from build123d import *

# Parameters (mm, degrees)
SKETCH013_W  = 32.5
SKETCH013_H  = 12.2
SKETCH013_R  = 1.35
PAD003_DEPTH = 1.2
SKETCH014_W  = 23
SKETCH014_H  = 12.2
PAD001_DEPTH = 1.4
PAD002_DEPTH = 6
SKETCH003_R  = 2.4
PAD005_DEPTH = 4.8
SKETCH016_W  = 23
SKETCH016_H  = 12.2
PAD004_DEPTH = 18.9
SKETCH012_W  = 3
SKETCH012_H  = 1
PAD008_DEPTH = 7


with BuildPart() as part:
    # Sketch013 → Pad003 (new body, symmetric)
    with BuildSketch(Plane.XY):
        Rectangle(SKETCH013_W, SKETCH013_H)
        with Locations((-13.8, 0)):
            Circle(SKETCH013_R, mode=Mode.SUBTRACT)
        with Locations((13.8, 0)):
            Circle(SKETCH013_R, mode=Mode.SUBTRACT)
    extrude(amount=PAD003_DEPTH, both=True)

    # Sketch014 → Pad001 (join)
    with BuildSketch(Plane.XY.offset(1.2)):
        Rectangle(SKETCH014_W, SKETCH014_H)
    extrude(amount=PAD001_DEPTH)

    # Sketch015 → Pad002 (join)
    with BuildSketch(Plane.XY.offset(2.6)):
        with BuildLine():
            ThreePointArc((-0.26712, 3.295988), (-11.5, 0), (-0.26712, -3.295988))
            ThreePointArc((0.490093, -2.839869), (0.058351, -2.979717), (-0.26712, -3.295988))
            ThreePointArc((0.490093, -2.839869), (3.1, 0), (0.490093, 2.839869))
            ThreePointArc((-0.26712, 3.295988), (0.058351, 2.979717), (0.490093, 2.839869))
        make_face()
    extrude(amount=PAD002_DEPTH)

    # Sketch003 → Pad005 (join)
    with BuildSketch(Plane.XY.offset(8.6)):
        with Locations((-5.4, 0)):
            Circle(SKETCH003_R)
    extrude(amount=PAD005_DEPTH)

    # Sketch016 → Pad004 (join)
    with BuildSketch(Plane(origin=(0, 0, -1.2), x_dir=(1, 0, 0), z_dir=(0, 0, -1))):
        Rectangle(SKETCH016_W, SKETCH016_H)
    extrude(amount=PAD004_DEPTH)

    # Sketch012 (on Face11 of Pad004) → Pad008 (join)
    with BuildSketch(Plane(origin=(-11.5, 0, 0), x_dir=(0, -1, 0), z_dir=(-1, 0, 0))):
        with Locations((0, -14.2)):
            Rectangle(SKETCH012_W, SKETCH012_H)
    extrude(amount=PAD008_DEPTH)


solid = part.part
Read the model definition and answer for the solid it produces. Units are mm, in the model's axes. A direction names the side the tool comes from. Coordinates: 2 decimals unless noted, no trailing zeros. Loops run counter-clockwise (first coordinate to the right, second up) from the corner with the lowest first, then second, coordinate; pieces in that order, holes last. Notation, with made-up numbers: (84.5, 87.25) -> (123.5, 87.25) arc R17 cw to (123.5, 96.25) -> close; hole circle Ø6 at (11.25, 44.25). An arc over 180 degrees is marked (long way). Write item = value, one per line. Start each with the question number.
1) The part is cut by section B-B, the plane x = 13.8. Determine the outline of the cut face in (y, z), plus the area to 3 significant figures.
2) Find the intervals of material crossed by L1, parallel to Y at x = -13.8, z = -0.05; L2, parallel to Z at x = -12, y = -1; L3, parallel to Z at x = 6.5, y = -5.5, in increasing order. Write a range as from..to.
3) The part is cut by section D-D, the plane x = 1.5. Determine the outline of the cut face in (y, z), plus the area to 3 significant figures.
4) For faces 4 (the face through (11.5, 0, 2)), 5 (the face through (-15, 0, -14.7)), 6 (the face through (-15, -1.5, -14)), 7 (the face through (5, 0, 2.6)), determine the directions among +Z, -Z, +X, -X, +Y, -Y from which every point of the face is accessible in a straight line to the end or side of a thin tool.
5) The part is cut by section A-A, the plane x = -13.8. Determine the outline of the cut face in (y, z), plus the area to 3 significant figures.
6) Given P1, Ø4, axis at x = 1.5, z = 10, coming from the -Y side; P2, Ø1.1, axis at y = 1.5, z = 2, coming from the -X side; P3, Ø4, axis at y = 1.5, z = 2, coming from the -X side, each flat-ended and moving along its own axis, determine where each tip first touches the part or whether it passes through.
7) The mould has two halves that part along Z. Classify faces 1 (the face through (-10, 5, 2.6)), 2 (the face through (-15, 0, -13.7)), 3 (the face through (-16.25, 0, 0)): pulls with the +Z half, pulls with the -Z half, needs draft (parallel to the pull), parting line crosses it, or undercut.
8) The part is cut by section C-C, the plane z = 4. Determine the outline of the cut face in (x, y).
Result:
q1.outline = (-6.1, -1.2) -> (-1.35, -1.2) -> (-1.35, 1.2) -> (-6.1, 1.2) -> close; (1.35, -1.2) -> (6.1, -1.2) -> (6.1, 1.2) -> (1.35, 1.2) -> close
q1.area = 22.8 mm²
q2.L1 = -6.1..-1.35, 1.35..6.1
q2.L2 = -14.7..-13.7, -1.2..1.2
q2.L3 = -20.1..2.6
q3.outline = (-6.1, -20.1) -> (6.1, -20.1) -> (6.1, 2.6) -> (2.56, 2.6) -> (2.56, 8.6) -> (-2.56, 8.6) -> (-2.56, 2.6) -> (-6.1, 2.6) -> close
q3.area = 308 mm²
q4.face_4 = +Z, +X, +Y, -Y
q4.face_5 = -Z, -X, +Y, -Y
q4.face_6 = -Z, -X, -Y
q4.face_7 = +Z, +X
q5.outline = (-6.1, -1.2) -> (-1.35, -1.2) -> (-1.35, 1.2) -> (-6.1, 1.2) -> close; (-1.5, -14.7) -> (1.5, -14.7) -> (1.5, -13.7) -> (-1.5, -13.7) -> close; (1.35, -1.2) -> (6.1, -1.2) -> (6.1, 1.2) -> (1.35, 1.2) -> close
q5.area = 25.8 mm²
q6.P1 = -2.97
q6.P2 = -11.5
q6.P3 = -16.25
q7.face_1 = pulls with the +Z half
q7.face_2 = undercut
q7.face_3 = needs draft
q8.outline = (-0.27, -3.3) arc R1 cw to (0.49, -2.84) arc R2.85 ccw to (0.49, 2.84) arc R1 cw to (-0.27, 3.3) arc R6.1 ccw (long way) to start
